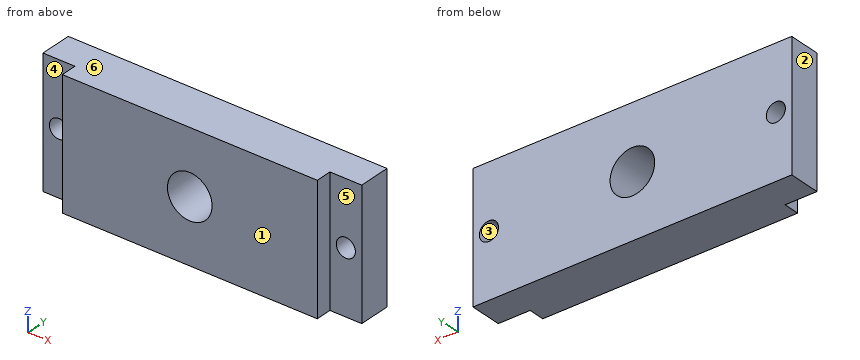
from build123d import *

# Parameters (mm, degrees)
EXTRUSION1_DEPTH        = 20
ESQUISSE2_R             = 3.5
ENL_V_MAT_EXTRU_1_DEPTH = 20
ESQUISSE3_R             = 1.5
ENL_V_MAT_EXTRU_2_DEPTH = 10


with BuildPart() as part:
    # Esquisse1 → Extrusion1 (new body)
    with BuildSketch(Plane.XY):
        Polygon((0, 0), (-50, 0), (-50, -5), (-45, -5), (-45, -7.5), (-5, -7.5), (-5, -5), (0, -5), align=None)
    extrude(amount=EXTRUSION1_DEPTH)

    # Esquisse2 → Enlèv. mat.-Extru.1 (cut)
    with BuildSketch(Plane(origin=(0, 0, 0), x_dir=(1, 0, 0), z_dir=(0, 1, 0))):
        with Locations(Location((-25, -10, 0), (0, 0, 180))):
            Circle(ESQUISSE2_R)
    extrude(amount=-ENL_V_MAT_EXTRU_1_DEPTH, mode=Mode.SUBTRACT)

    # Esquisse3 → Enlèv. mat.-Extru.2 (cut)
    with BuildSketch(Plane.XZ.offset(5)):
        with Locations(Location((-47.5, 10, 0), (0, 0, 270))):
            Circle(ESQUISSE3_R)
        with Locations((-2.5, 10)):
            Circle(ESQUISSE3_R)
    extrude(amount=-ENL_V_MAT_EXTRU_2_DEPTH, mode=Mode.SUBTRACT)


solid = part.part
Can you work these out from the model? Positions are in its coordinate system, mm. Face numbers are marked on the shaded views. A direction names the side the tool comes from. Coordinates: 2 decimals unless noted, no trailing zeros. Order: outer loops, then holes, each group sorted by start corner. A loop starts at its lowest first (then second) coordinate and runs counter-clockwise, first axis right, second up. Notation, with made-up numbers: (74, 50.25) - (94, 50.25) arc R35 cw to (94, 87.25) - close; hole circle Ø4 at (14.25, 8.25). An arc over 180 degrees is marked (long way). Answer as a JSON object with one key per item and string values. Group by question number.
Q1. I need wall thicknesses on line 1 (Z direction, x = -25, y = -2.5); line 2 (Z direction, x = -2.5, y = -3.6); line 3 (X direction, y = -4, z = 9.25). Which ranges of each line are inside material? Lowest first, please. Write a range as from..to.
Q2. Imagine slicing it at B-B (z = 10). Please give me the cut outline in (x, y).
Q3. Imagine slicing it at A-A (x = -25). Please give me the cut outline in (y, z), and give its area (3 significant figures).
Q4. Will these pins go through, and if not, where does the flat tip stop? P1, Ø2, axis at y = -6.5, z = 12.5, coming from the +X side; P2, Ø1.5, axis at x = -3, z = 5.5, coming from the -Y side.
Q5. Imagine slicing it at D-D (z = 8). Please give me the cut outline in (x, y), and give its area (3 significant figures).
Q6. We'd pull the mould along X, two halves only. Please class the marked faces 1, 2 and 3: +X half, -X half, draft (parallel to the pull), parting line (faces both ways), or undercut.
Q7. Imagine slicing it at C-C (y = -4.25). Please give me the cut outline in (x, z).
Q8. On a 3-axis mill with a long thin cutter (end or side, diameter ignored), from which of +Z, -Z, +X, -X, +Y, -Y can I reach the whole of each face in a straight line? I mean the marked faces 4, 5 and 6. Say none if no direction works.
Determined:
{
 "1": {"line 1": "z = 0..6.5, 13.5..20", "line 2": "z = 0..8.5, 11.5..20", "line 3": "x = -50..-48.8, -46.2..-28.42, -21.58..-3.8, -1.2..0"},
 "2": {"outline": "(-50, -5) - (-49, -5) - (-49, 0) - (-50, 0) - close; (-46, -5) - (-45, -5) - (-45, -7.5) - (-28.5, -7.5) - (-28.5, 0) - (-46, 0) - close; (-21.5, -7.5) - (-5, -7.5) - (-5, -5) - (-4, -5) - (-4, 0) - (-21.5, 0) - close; (-1, -5) - (0, -5) - (0, 0) - (-1, 0) - close"},
 "3": {"outline": "(-7.5, 0) - (0, 0) - (0, 6.5) - (-7.5, 6.5) - close; (-7.5, 13.5) - (0, 13.5) - (0, 20) - (-7.5, 20) - close", "area": "97.5 mm2"},
 "4": {"P1": "stops at x = -5", "P2": "stops at y = -5"},
 "5": {"outline": "(-50, -5) - (-45, -5) - (-45, -7.5) - (-27.87, -7.5) - (-27.87, 0) - (-50, 0) - close; (-22.13, -7.5) - (-5, -7.5) - (-5, -5) - (0, -5) - (0, 0) - (-22.13, 0) - close", "area": "307 mm2"},
 "6": {"face 1": "draft", "face 2": "-X half", "face 3": "undercut"},
 "7": {"outline": "(-50, 0) - (0, 0) - (0, 20) - (-50, 20) - close; hole circle Ø3 at (-47.5, 10); hole circle Ø7 at (-25, 10); hole circle Ø3 at (-2.5, 10)"},
 "8": {"face 4": "+Z, -Z, -X, -Y", "face 5": "+Z, -Z, +X, -Y", "face 6": "+Z, +X, -X, +Y, -Y"}
}
